Here's how the part is built. I have some questions about the finished solid (model axes, mm). A direction names the side the tool comes from. Round coordinates to 2 decimals unless told otherwise and drop trailing zeros. Write each loop counter-clockwise with the first axis right and the second up, starting at its lowest first coordinate (ties: lowest second). Pieces come first, ordered by that corner, then holes. Notation, with made-up numbers: (8.25, 67.5) - (43.25, 67.5) arc R34 ccw to (43.25, 100.5) - close; hole circle Ø10 at (55.5, -4.75). An arc over 180 degrees is marked (long way). One line per item, written item: value. Start each with the question number.
Item 1: Imagine slicing it at C-C, the plane x = -2.5. Please give me the cut outline in (y, z), then the cut area to 3 significant figures.
Item 2: Imagine slicing it at B-B, the plane y = 2. Please give me the cut outline in (x, z).
Item 3: For faces 1 (the face through (-3.905, 18.325, -0.867)), 2 (the face through (-5.515, 0.162, -3.221)), which set-ups out of +Z, -Z, +X, -X, +Y, -Y let a thin tool reach every point of the face, with its end or its side?
Item 4: For P1, Ø5, axis at x = -4.5, y = 11, coming from the +Z side; P2, Ø3, axis at x = -0.5, y = 12, coming from the +Z side; P3, Ø1, axis at x = 3, y = 16.5, coming from the +Z side, each with a flat end and sliding along its axis, tell me the tip position at first contact or that it passes through.
Item 5: Imagine slicing it at A-A, the plane z = 0. Please give me the cut outline in (x, y).
Item 6: If I drill on line 1 (Y direction, x = -3.25, z = 4.75); line 2 (X direction, y = 27.5, z = 0); line 3 (X direction, y = 18, z = 1), over which ranges is the centre line in solid material (lowest first)?
Item 7: Imagine slicing it at D-D, the plane y = 14.5. Please give me the cut outline in (x, z).
```python
from build123d import *

# Parameters (mm, degrees)
BOSS_EXTRUDE1_DEPTH = 6
SKETCH6_R           = 4
BOSS_EXTRUDE2_DEPTH = 25


with BuildPart() as part:
    # Sketch1 → Boss-Extrude1 (new body)
    with BuildSketch(Plane(origin=(0, 0, 0), x_dir=(1, 0, 0), z_dir=(0, 1, 0))):
        Polygon((6.062177826, 3.5), (0, 7), (-6.062177826, 3.5), (-6.062177826, -3.5), (0, -7), (6.062177826, -3.5), align=None)
    extrude(amount=BOSS_EXTRUDE1_DEPTH)

    # Sketch5 → Cut-Revolve5 (revolve, cut)
    with BuildSketch(Plane(origin=(0, 0, 0), x_dir=(0, 0, -1), z_dir=(1, 0, 0))):
        Polygon((5.527622028, -0.407756563), (7.359129526, 0.805892984), (7.359129526, -0.407756563), align=None)
    revolve(axis=Axis((0, 0, 0), (0, 1, 0)), mode=Mode.SUBTRACT)

    # Sketch6 → Boss-Extrude2 (add)
    with BuildSketch(Plane(origin=(0, 6, 0), x_dir=(1, 0, 0), z_dir=(0, 1, 0))):
        with Locations(Location((0, 0, 0), (0, 0, 270))):  # turned: the seam where the file's is
            Circle(SKETCH6_R)
    extrude(amount=BOSS_EXTRUDE2_DEPTH)


solid = part.part
```
Values follow:
1. outline: (0, -5.56) - (6, -5.56) - (6, -3.12) - (31, -3.12) - (31, 3.12) - (6, 3.12) - (6, 5.56) - (0, 5.56) - close
1. area: 223 mm^2
2. outline: (-6.06, -3.5) - (0, -7) - (6.06, -3.5) - (6.06, 3.5) - (0, 7) - (-6.06, 3.5) - close
3. face 1: +Y
3. face 2: -Z, -X, -Y
4. P1: stops at z = 3.46
4. P2: stops at z = 4
4. P3: stops at z = 3.12
5. outline: (-6.06, 0) - (6.06, 0) - (6.06, 6) - (4, 6) - (4, 31) - (-4, 31) - (-4, 6) - (-6.06, 6) - close
6. line 1: y = 0 to 6
6. line 2: x = -4 to 4
6. line 3: x = -3.87 to 3.87
7. outline: circle Ø8 at (0, 0)
